Autodesk Inventor part; units mm, degrees
ref_plane "YZ Plane" through (0, 0, 0) normal (1, 0, 0) x (0, 1, 0)
ref_plane "XZ Plane" through (0, 0, 0) normal (0, 1, 0) x (-1, 0, 0)
ref_plane "XY Plane" through (0, 0, 0) normal (0, 0, 1) x (1, 0, 0)
sketch "Sketch1" plane through (0, 0, 0) normal (0, 1, 0) x (-1, 0, 0)
  line L0 (-100, 284.5) -> (-100, 98)
  line L1 (-100, 98) -> (140, 98)
  line L2 (140, 98) -> (140, -98)
  line L3 (140, -98) -> (-100, -98)
  line L4 (-100, -98) -> (-100, -284.5)
  line L5 (-100, 284.5) -> (144, 284.5)
  line L6 (144, 284.5) -> (144, 240.5)
  line L7 (144, 240.5) -> (131.5, 240.5)
  line L8 (131.5, 240.5) -> (131.5, 148)
  line L9 (131.5, 148) -> (183.5, 148)
  line L10 (183.5, 148) -> (203.5, 98)
  line L11 (-100, -284.5) -> (144, -284.5)
  line L12 (144, -284.5) -> (144, -240.5)
  line L13 (144, -240.5) -> (131.5, -240.5)
  line L14 (131.5, -240.5) -> (131.5, -148)
  line L15 (131.5, -148) -> (183.5, -148)
  line L16 (183.5, -148) -> (203.5, -98)
  line L17 (203.5, 98) -> (203.5, -98)
  line L18 (-38, 240.5) -> (-38, 148)
  line L19 (-38, 148) -> (87, 148)
  line L20 (87, 148) -> (87, 240.5)
  line L21 (87, 240.5) -> (-38, 240.5)
  line L22 (-38, -148) -> (-38, -240.5)
  line L23 (-38, -240.5) -> (87, -240.5)
  line L24 (87, -240.5) -> (87, -148)
  line L25 (87, -148) -> (-38, -148)
  point P0 (0, 0)
  point P1 (140, 0)
  dimension "d4" = 196
  dimension "d8" = 244
  dimension "d9" = 44
  dimension "d10" = 12.5
  dimension "d12" = 52
  dimension "d13" = 50
  dimension "d14" = 20
  dimension "d17" = 12.5
  dimension "d19" = 52
  dimension "d20" = 50
  dimension "d21" = 20
  dimension "d23" = 92.5
  dimension "d24" = 125
  dimension "d25" = 62
  dimension "d26" = 44
  dimension "d27" = 92.5
  dimension "d28" = 125
  dimension "d29" = 62
  dimension "d30" = 44
  dimension "d64" = 240
  dimension "d65" = 240
  dimension "d66" = 50
  dimension "d69" = 92.5
  dimension "d70" = 196
  dimension "d76" = 44
extrude "Extrusion1" add sketch "Sketch1" along normal blind 6.5
sketch "Sketch3" plane through (0, 0, 0) normal (0, -1, 0) x (1, 0, 0)
  line L0 (-87, -148) -> (38, -148) construction
  line L1 (38, -148) -> (38, -240.5) construction
  line L2 (38, -240.5) -> (-87, -240.5) construction
  line L3 (-87, -240.5) -> (-87, -148) construction
  line L4 (-87, 240.5) -> (38, 240.5) construction
  line L5 (38, 240.5) -> (38, 148) construction
  line L6 (38, 148) -> (-87, 148) construction
  line L7 (-87, 148) -> (-87, 240.5) construction
  line L8 (100, 284.5) -> (100, 98) construction
  line L9 (-144, 284.5) -> (100, 284.5) construction
  line L10 (-144, 240.5) -> (-144, 284.5) construction
  line L11 (-131.5, 240.5) -> (-144, 240.5) construction
  line L12 (-131.5, 148) -> (-131.5, 240.5) construction
  line L13 (-183.5, 148) -> (-131.5, 148) construction
  line L14 (-203.5, 98) -> (-183.5, 148) construction
  line L15 (-203.5, -98) -> (-203.5, 98) construction
  line L16 (-183.5, -148) -> (-203.5, -98) construction
  line L17 (-131.5, -148) -> (-183.5, -148) construction
  line L18 (-131.5, -240.5) -> (-131.5, -148) construction
  line L19 (-144, -240.5) -> (-131.5, -240.5) construction
  line L20 (-144, -284.5) -> (-144, -240.5) construction
  line L21 (100, -284.5) -> (-144, -284.5) construction
  line L22 (100, -98) -> (100, -284.5) construction
  line L23 (-140, -98) -> (100, -98) construction
  line L24 (-140, 98) -> (-140, -98) construction
  line L25 (100, 98) -> (-140, 98) construction
  line L26 (100, -98) -> (100, -284.5)
  line L27 (-131.5, -148) -> (-183.5, -148)
  line L28 (100, -98) -> (-203.5, -98)
  line L29 (-140, -98) -> (100, -98)
  line L30 (-183.5, -148) -> (-203.5, -98)
  line L31 (-183.5, -148) -> (100, -148)
  line L32 (100, -98) -> (100, -284.5)
  line L33 (100, -98) -> (100, -148)
  line L34 (100, 284.5) -> (100, 98)
  line L35 (-203.5, -98) -> (-203.5, 98)
  line L36 (100, 98) -> (-203.5, 98)
  line L37 (-203.5, 98) -> (-183.5, 148)
  line L38 (100, 148) -> (100, 98)
  line L39 (-183.5, 148) -> (-131.5, 148)
  line L40 (100, 148) -> (-183.5, 148)
  line L41 (-183.5, -148) -> (-203.5, -98)
  line L42 (-203.5, -98) -> (-183.5, -148)
  point P0 (0, 0)
extrude "Extrusion3" add sketch "Sketch3" along normal blind 38
sketch "Sketch4" plane through (0, 0, 0) normal (0, -1, 0) x (1, 0, 0)
  line L0 (-203.5, -98) -> (-203.5, 98)
  line L1 (-140, 98) -> (-203.5, 98)
  line L2 (-203.5, 98) -> (-140, 98)
  line L3 (-140, 98) -> (-140, -98)
  line L4 (-140, 98) -> (-140, -98)
  line L5 (-140, -98) -> (-203.5, -98)
  line L6 (-203.5, -98) -> (-203.5, 98)
  point P0 (0, 0)
extrude "Extrusion4" add sketch "Sketch4" along normal blind 38
sketch "Sketch5" plane through (0, 6.5, 0) normal (0, 1, 0) x (1, 0, 0)
  line L0 (38, 148) -> (-87, 148) construction
  line L1 (-87, 148) -> (-87, 240.5) construction
  line L2 (-87, 240.5) -> (38, 240.5) construction
  line L3 (38, 240.5) -> (38, 148) construction
  line L4 (38, -240.5) -> (-87, -240.5) construction
  line L5 (-87, -240.5) -> (-87, -148) construction
  line L6 (-87, -148) -> (38, -148) construction
  line L7 (38, -148) -> (38, -240.5) construction
  line L8 (100, -284.5) -> (100, -98) construction
  line L9 (100, -98) -> (-140, -98) construction
  line L10 (-140, -98) -> (-140, 98) construction
  line L11 (-140, 98) -> (100, 98) construction
  line L12 (100, 98) -> (100, 284.5) construction
  line L13 (100, 284.5) -> (-144, 284.5) construction
  line L14 (-144, 284.5) -> (-144, 240.5) construction
  line L15 (-144, 240.5) -> (-131.5, 240.5) construction
  line L16 (-131.5, 240.5) -> (-131.5, 148) construction
  line L17 (-131.5, 148) -> (-183.5, 148) construction
  line L18 (-183.5, 148) -> (-203.5, 98) construction
  line L19 (-203.5, 98) -> (-203.5, -98) construction
  line L20 (-203.5, -98) -> (-183.5, -148) construction
  line L21 (-183.5, -148) -> (-131.5, -148) construction
  line L22 (-131.5, -148) -> (-131.5, -240.5) construction
  line L23 (-131.5, -240.5) -> (-144, -240.5) construction
  line L24 (-144, -240.5) -> (-144, -284.5) construction
  line L25 (-144, -284.5) -> (100, -284.5) construction
  line L26 (-140, -98) -> (-140, 98)
  line L27 (-140, -98) -> (-140, 98)
  line L28 (-140, 98) -> (100, 98)
  line L29 (-140, 98) -> (38, 98)
  line L30 (38, 240.5) -> (38, 148)
  line L31 (38, 98) -> (38, 148)
  line L32 (-87, 240.5) -> (-87, 148)
  line L33 (-87, 148) -> (-87, 240.5)
  line L34 (-131.5, 240.5) -> (-131.5, 148)
  line L35 (-131.5, 148) -> (-131.5, 240.5)
  line L36 (38, 148) -> (-87, 148)
  line L37 (38, 148) -> (-87, 148)
  line L38 (-131.5, 148) -> (-183.5, 148)
  line L39 (-131.5, 148) -> (-183.5, 148)
  line L40 (-183.5, 148) -> (-203.5, 98)
  line L41 (-203.5, 98) -> (-203.5, -98)
  line L42 (-203.5, 98) -> (-203.5, -98)
  line L43 (100, -148) -> (-183.5, -148)
  line L44 (-203.5, -98) -> (-183.5, -148)
  line L45 (-183.5, -148) -> (-131.5, -148)
  line L46 (-131.5, -148) -> (-131.5, -240.5)
  line L47 (-131.5, -148) -> (-131.5, -240.5)
  line L48 (-87, -240.5) -> (-87, -148)
  line L49 (-87, -240.5) -> (-87, -148)
  line L50 (-87, -148) -> (38, -148)
  line L51 (-140, -98) -> (100, -98)
  line L52 (38, -98) -> (38, -148)
  line L53 (38, -98) -> (-140, -98)
  line L54 (38, -148) -> (38, -240.5)
  line L55 (38, -240.5) -> (38, -284.5)
  line L56 (-144, -284.5) -> (100, -284.5)
  line L57 (-144, -240.5) -> (-144, -284.5)
  line L58 (-144, -284.5) -> (-144, -240.5)
  line L59 (-144, -240.5) -> (-131.5, -240.5)
  line L60 (38, -240.5) -> (-87, -240.5)
  line L61 (-87, -240.5) -> (38, -240.5)
  line L62 (38, -284.5) -> (-144, -284.5)
  line L63 (38, 240.5) -> (-87, 240.5)
  line L64 (-87, 240.5) -> (38, 240.5)
  line L65 (38, 240.5) -> (38, 284.5)
  line L66 (100, 284.5) -> (-144, 284.5)
  line L67 (-144, 284.5) -> (38, 284.5)
  line L68 (-144, 284.5) -> (-144, 240.5)
  line L69 (-144, 284.5) -> (-144, 240.5)
  line L70 (-144, 240.5) -> (-131.5, 240.5)
  point P0 (0, 0)
extrude "Extrusion5" cut sketch "Sketch5" against normal blind 3.25 contours L51 L52 L43 L44 L41 L40 L38 L34 L70 L68 L66 L65 L63 L32 L36 L31 L28 L26 | L48 L60 L55 L56 L57 L59 L46 L43
sketch "Sketch6" plane through (0, 3.25, 0) normal (0, 1, 0) x (1, 0, 0)
  line L0 (-87, 148) -> (38, 148) construction
  line L1 (-87, 240.5) -> (-87, 148) construction
  line L2 (38, 240.5) -> (-87, 240.5) construction
  line L3 (38, 284.5) -> (38, 240.5) construction
  line L4 (-144, 284.5) -> (38, 284.5) construction
  line L5 (-144, 240.5) -> (-144, 284.5) construction
  line L6 (-131.5, 240.5) -> (-144, 240.5) construction
  line L7 (-131.5, 148) -> (-131.5, 240.5) construction
  line L8 (-183.5, 148) -> (-131.5, 148) construction
  line L9 (-203.5, 98) -> (-183.5, 148) construction
  line L10 (-203.5, -98) -> (-203.5, 98) construction
  line L11 (-183.5, -148) -> (-203.5, -98) construction
  line L12 (-131.5, -148) -> (-183.5, -148) construction
  line L13 (-131.5, -240.5) -> (-131.5, -148) construction
  line L14 (-144, -240.5) -> (-131.5, -240.5) construction
  line L15 (-144, -284.5) -> (-144, -240.5) construction
  line L16 (38, -284.5) -> (-144, -284.5) construction
  line L17 (38, -240.5) -> (38, -284.5) construction
  line L18 (-87, -240.5) -> (38, -240.5) construction
  line L19 (-87, -148) -> (-87, -240.5) construction
  line L20 (38, -148) -> (-87, -148) construction
  line L21 (38, -98) -> (38, -148) construction
  line L22 (-140, -98) -> (38, -98) construction
  line L23 (-140, 98) -> (-140, -98) construction
  line L24 (38, 98) -> (-140, 98) construction
  line L25 (38, 148) -> (38, 98) construction
  line L26 (38, -149) -> (-87, -149)
  line L27 (38, -148) -> (-87, -148)
  line L28 (-87, -148) -> (-87, -240.5)
  line L29 (-131.5, -240.5) -> (-87, -240.5)
  line L30 (-131.5, -148) -> (-131.5, -240.5)
  line L31 (-131.5, -240.5) -> (-131.5, -148)
  line L32 (100, -148) -> (-183.5, -148)
  line L33 (-131.5, -148) -> (-183.5, -148)
  line L34 (-203.5, -98) -> (-203.5, 98)
  line L35 (-183.5, -148) -> (-203.5, -98)
  line L36 (-203.5, -98) -> (-203.5, 98)
  line L37 (-203.5, 98) -> (-183.5, 148)
  line L38 (-131.5, 240.5) -> (-131.5, 148)
  line L39 (-183.5, 148) -> (100, 148)
  line L40 (-131.5, 148) -> (-183.5, 148)
  line L41 (-144, 240.5) -> (-131.5, 240.5)
  line L42 (-131.5, 148) -> (-131.5, 240.5)
  line L43 (-131.5, 240.5) -> (-87, 240.5)
  line L44 (-87, 240.5) -> (-87, 148)
  line L45 (-87, 148) -> (-87, 240.5)
  line L46 (38, 148) -> (38, 240.5)
  line L47 (-87, 148) -> (38, 148)
  line L48 (38, 148) -> (38, 98)
  line L49 (38, 148) -> (38, 98)
  line L50 (100, 98) -> (-140, 98)
  line L51 (38, 98) -> (-140, 98)
  line L52 (-140, 98) -> (-140, -98)
  line L53 (-140, 98) -> (-140, -98)
  line L54 (-140, -98) -> (38, -98)
  line L55 (38, -98) -> (38, -284.5)
  line L56 (38, -148) -> (38, -98)
  point P0 (0, 0)
extrude "Extrusion6" add sketch "Sketch6" against normal blind 6.25 contours L28 L29 L30 L32 | L27 L32 L35 L34 L37 L39 L48 L50 L52 L54 L55 | L39 L38 L43 L44
extrude "Extrusion7" cut sketch "Sketch6" against normal blind 3.25 contours L28 L29 L30 L32 | L27 L32 L35 L34 L37 L39 L48 L50 L52 L54 L55 | L39 L38 L43 L44
sketch "Sketch7" plane through (0, 0, 0) normal (0, -1, 0) x (1, 0, 0)
  line L0 (38, 148) -> (100, 148)
  line L1 (93.5, 148) -> (100, 148)
  line L2 (100, 284.5) -> (100, 148)
  line L3 (100, 285) -> (100, 148)
  line L4 (-144, 284.5) -> (100, 284.5)
  line L5 (-144, 240.5) -> (-144, 284.5)
  line L6 (100, 284.5) -> (-144, 284.5)
  line L7 (-144, 240.5) -> (-144, 284.5)
  line L8 (93.5, 280) -> (93.5, 148)
  line L9 (-144, 240.5) -> (38, 240.5)
  line L10 (-141, 240.5) -> (-141, 280)
  line L11 (-141, 280) -> (93.5, 280)
  line L12 (-141, 240.5) -> (-144, 240.5)
  line L13 (-573.3935, 0) -> (506.825, 0) construction
  line L14 (93.5, -148) -> (100, -148)
  line L15 (100, -284.5) -> (100, -148)
  line L16 (-144, -284.5) -> (100, -284.5)
  line L17 (-144, -240.5) -> (-144, -284.5)
  line L18 (100, -284.5) -> (-144, -284.5)
  line L19 (93.5, -280) -> (93.5, -148)
  line L20 (-141, -240.5) -> (-141, -280)
  line L21 (38, -240.5) -> (38, -148) construction
  line L22 (38, -240.5) -> (-144, -240.5) construction
  line L23 (-141, -240.5) -> (-144, -240.5)
  line L24 (-141, -280) -> (93.5, -280)
  line L25 (-144, -240.5) -> (-144, -284.5)
  line L26 (100, -98) -> (100, -284.5)
  line L27 (100, -148) -> (100, -284.5)
  point P0 (0, 0)
  dimension "d85" = 3
  dimension "d86" = 4.5
  dimension "d87" = 6.5
extrude "Extrusion8" add sketch "Sketch7" along normal blind 35.5
sketch "Sketch8" plane through (100, 6.5, 284.5) normal (1, 0, 0) x (0, 0, -1)
  line L0 (142.5, -38.5) -> (142.5, -12.5)
  line L1 (142.5, -12.5) -> (180.5, -12.5)
  line L2 (180.5, -38.5) -> (142.5, -38.5)
  line L3 (180.5, -12.5) -> (180.5, -38.5)
  line L4 (186.5, -44.5) -> (186.5, 0)
  line L5 (186.5, -44.5) -> (136.5, -44.5)
  line L6 (136.5, -42) -> (136.5, -44.5)
  line L7 (0, 0) -> (186.5, 0)
  line L8 (285, -82.0279) -> (285, 56.7605) construction
  line L9 (427.5, -38.5) -> (427.5, -12.5)
  line L10 (427.5, -12.5) -> (389.5, -12.5)
  line L11 (389.5, -38.5) -> (427.5, -38.5)
  line L12 (389.5, -12.5) -> (389.5, -38.5)
  point P0 (284.5, -6.5)
  point P1 (136.5, -6.5)
  dimension "d90" = 6
  dimension "d91" = 6
  dimension "d92" = 6
  dimension "d93" = 12.5
extrude "Extrusion9" cut sketch "Sketch8" against normal through all
extrude "Extrusion10" add sketch "Sketch8" against normal blind 6.5
properties part number "battlebotupperframe"
Could you check a few things on this model? Use its own coordinates, in mm. A direction names the side the tool comes from. Round coordinates to 2 decimals unless told otherwise and drop trailing zeros. Write each loop counter-clockwise with the first axis right and the second up, starting at its lowest first coordinate (ties: lowest second). Pieces come first, ordered by that corner, then holes. Notation, with made-up numbers: (70.5, -20.5) - (76.5, -20.5) arc R5 cw to (76.5, -11.5) - close; hole circle Ø8 at (56, 66.25). An arc over 180 degrees is marked (long way). Put each result on its own line as item: value. Start each with the question number.
(1) Will these pins go through, and if not, where does the flat tip stop? pin 1 (19.5 mm diameter, centred on y = -13.5, z = 256.5, fed in from -X); pin 2 (1 mm diameter, centred on x = -171.5, y = -9, fed in from +Z); pin 3 (8 mm diameter, centred on x = -141, z = -69, fed in from +Y).
(2) For faces 1 (the flat face through (32, -35.5, -282)), 2 (the flat face through (-140, -19, 1)), 3 (the flat face through (-44, -19, -143)), 4 (the flat face through (93.5, -18, 215)), 5 (the flat face through (-144, -16, -263)), which set-ups out of +Z, -Z, +X, -X, +Y, -Y let a thin tool reach every point of the face, with its end or its side?
(3) Thinking about a two-plate mould opening in Z: for faces 6 (the flat face through (-54, 3.25, 262)), 7 (the flat face through (-20, -15, -284.5)), 8 (the flat face through (-44, -19, 148)), which applies, released by +Z, released by -Z, zero draft, split by the parting line, or undercut?
(4) I want a section at A-A, the plane x = 50. Please give me the cut outline in (y, z), plus the area to 3 significant figures.
(5) I want a section at B-B, the plane z = 183. Please give me the cut outline in (x, y).
(6) I need wall thicknesses on probe 1 along Z at (x, y) = (-122.5, -14); probe 2 along Z at (x, y) = (83, -35); probe 3 along X at (y, z) = (-17, -245.5). Which ranges of each line are inside material? Lowest first, please.
Here are the results:
1. pin 1: stops at x = -144
1. pin 2: stops at z = 148
1. pin 3: stops at y = 0
2. face 1: -Z, +X, -X, -Y
2. face 2: +X, +Y, -Y
2. face 3: -X
2. face 4: -Y
2. face 5: -Z, -X, +Y, -Y
3. face 6: zero draft
3. face 7: released by -Z
3. face 8: undercut
4. outline: (-38, -148) - (0, -148) - (0, -280) - (-35.5, -280) - (-35.5, -284.5) - (6.5, -284.5) - (6.5, -98) - (-38, -98) - close; (-38, 98) - (6.5, 98) - (6.5, 284.5) - (-35.5, 284.5) - (-35.5, 280) - (0, 280) - (0, 148) - (-38, 148) - close; hole (-32, -143) - (-6, -143) - (-6, -105) - (-32, -105) - close; hole (-32, 104) - (-6, 104) - (-6, 142) - (-32, 142) - close
4. area: 4,570 mm^2
5. outline: (-131.5, -3) - (-87, -3) - (-87, 0) - (-131.5, 0) - close; (38, 0) - (93.5, 0) - (93.5, -35.5) - (100, -35.5) - (100, 6.5) - (38, 6.5) - close
6. probe 1: z = -284.5 to -280, -148 to -143, -105 to -98, 98 to 104, 142 to 148, 280 to 284.5
6. probe 2: z = -284.5 to -280, -148 to -98, 98 to 148, 280 to 284.5
6. probe 3: x = -144 to -141, 93.5 to 100
